from build123d import *

# Parameters (mm, degrees)
SKETCH1_W           = 64.77
SKETCH1_H           = 6.35
SKETCH1_R           = 1.75
BOSS_EXTRUDE1_DEPTH = 6.35
BOSS_EXTRUDE2_START = -31.75
SKETCH2_R           = 3.175
SKETCH2_R_2         = 1.75
BOSS_EXTRUDE2_DEPTH = 25.4


with BuildPart() as part:
    # Sketch1 → Boss-Extrude1 (new body)
    with BuildSketch(Plane(origin=(0, 0, 0), x_dir=(1, 0, 0), z_dir=(0, 1, 0))):
        with Locations((32.385, 3.175)):
            Rectangle(SKETCH1_W, SKETCH1_H)
        with Locations(Location((3.81, 3.175, 0), (0, 0, 270))):
            Circle(SKETCH1_R, mode=Mode.SUBTRACT)
        with Locations(Location((60.96, 3.175, 0), (0, 0, 270))):
            Circle(SKETCH1_R, mode=Mode.SUBTRACT)
    extrude(amount=-BOSS_EXTRUDE1_DEPTH)

    # Sketch2 → Boss-Extrude2 (add)
    with BuildSketch(Plane.XZ.offset(6.35).offset(BOSS_EXTRUDE2_START)):
        with Locations(Location((3.81, -3.175, 0), (0, 0, 270))):
            Circle(SKETCH2_R)
        with Locations(Location((3.81, -3.175, 0), (0, 0, 90))):
            Circle(SKETCH2_R_2, mode=Mode.SUBTRACT)
    extrude(amount=BOSS_EXTRUDE2_DEPTH)


solid = part.part
Design review of the part built by this model. Coordinates are the model's own, in mm. A direction names the side the tool comes from. Coordinates: 2 decimals unless noted, no trailing zeros. Loops run counter-clockwise (first coordinate to the right, second up) from the corner with the lowest first, then second, coordinate; pieces in that order, holes last. Notation, with made-up numbers: M 82.25,51 L 99.25,51 A32 ccw 99.25,77 Z; hole C 48,14.5 d8. An arc over 180 degrees is marked long. Answer as CSV lines item,"result".
Item 1: Add section C-C on y = 23. State the section outline as (x, z) points (3 decimals).
Answer list:
outline,"C 3.81,-3.175 d6.35; hole C 3.81,-3.175 d3.5"
Item 2: Add section D-D on x = 36.5. State the section outline as (y, z) points.
Answer list:
outline,"M -6.35,-6.35 L 0,-6.35 L 0,0 L -6.35,0 Z"
Item 3: Machinability: for faces 5 (the face through (0.48, 0, -3.19)), 6 (the face through (2, 25.4, -5)), 7 (the face through (0.993, 12.878, -4.64)), which of the approach directions +Z, -Z, +X, -X, +Y, -Y give a long, thin tool a straight path to every point of the face, cutting with its end or side? Answer none if there is none.
Answer list:
face 5,"-X, +Y"
face 6,"+Z, -Z, +X, -X, +Y"
face 7,"+Y"
Item 4: The part is to be moulded in two halves that separate along X. For faces 1 (the face through (5.52, 9.75, -3.55)), 2 (the face through (64.77, -3, -3)), 3 (the face through (59.25, -3.13, -3.55)), 4 (the face through (32, -6.35, -3)), say which applies: pulls with the +X half, pulls with the -X half, needs draft (parallel to the pull), parting line crosses it, or undercut.
Answer list:
face 1,"undercut"
face 2,"pulls with the +X half"
face 3,"undercut"
face 4,"needs draft"
Item 5: For P1, Ø1.9, axis at x = 24.5, z = -4, coming from the +Y side; P2, Ø1.5, axis at y = 19.5, z = -5, coming from the +X side; P3, Ø1.9, axis at x = 2.5, z = -3, coming from the +Y side; P4, Ø1, axis at y = 14.5, z = -3, coming from the -X side (3 decimals), all flat-tipped, find the tip position at first contact; note any pin that passes through.
Answer list:
P1,"y = 0"
P2,"x = 6.8"
P3,"y = 25.4"
P4,"x = 0.635"
Item 6: Add section A-A on x = 60.96. State the section outline as (y, z) points (3 decimals), plus the area to 3 significant figures.
Answer list:
outline,"M -6.35,-6.35 L 0,-6.35 L 0,-4.925 L -6.35,-4.925 Z; M -6.35,-1.425 L 0,-1.425 L 0,0 L -6.35,0 Z"
area,"18.1 mm²"
Item 7: For probe 1 along X at (y, z) = (-1, -2); probe 2 along X at (y, z) = (-3.5, -4.5); probe 3 along X at (y, z) = (22.5, -3), list the stretches that pass through material, from the lowest coordinate up.
Answer list:
probe 1,"0 to 2.51, 5.11 to 59.66, 62.26 to 64.77"
probe 2,"0 to 2.67, 4.95 to 59.82, 62.1 to 64.77"
probe 3,"0.64 to 2.07, 5.55 to 6.98"
Item 8: Add section B-B on z = -3.25. State the section outline as (x, y) points, plus the area to 3 significant figures.
Answer list:
outline,"M 0,-6.35 L 2.06,-6.35 L 2.06,25.4 L 0.64,25.4 L 0.64,0 L 0,0 Z; M 5.56,-6.35 L 59.21,-6.35 L 59.21,0 L 6.98,0 L 6.98,25.4 L 5.56,25.4 Z; M 62.71,-6.35 L 64.77,-6.35 L 64.77,0 L 62.71,0 Z"
area,"439 mm²"
